from build123d import *

# Parameters (mm, degrees)
SKETCH1_R                    = 3.556
BOSS_EXTRUDE1_DEPTH          = 3.556
F_30_0_1285_DIAMETER_HOLE1_D = 3.2639
CHAMFER2_SIZE                = 0.381
F_65_0_035_DIAMETER_HOLE2_D  = 0.889
F_6_32_TAPPED_HOLE1_D        = 2.7051
F_6_32_TAPPED_HOLE1_DEPTH    = 5.7912
F_6_32_TAPPED_HOLE1_TIP      = 0.81269403


with BuildPart() as part:
    # Sketch1 → Boss-Extrude1 (new, symmetric)
    with BuildSketch(Plane(origin=(0, 0, 0), x_dir=(0, 0, -1), z_dir=(1, 0, 0))):
        Circle(SKETCH1_R)
    extrude(amount=BOSS_EXTRUDE1_DEPTH, both=True)

    # #30 (0.1285) Diameter Hole1 (through all)
    with Locations(Plane(origin=(3.556, 0, 0), x_dir=(0, 0, -1), z_dir=(1, 0, 0))):
        with Locations((0, 0)):
            Hole(F_30_0_1285_DIAMETER_HOLE1_D / 2)

    # Chamfer2
    chamfer2_edges = [part.edges().sort_by_distance(p)[0] for p in [
        (-3.556, 0, 3.556),
        (3.556, 0, 3.556),
    ]]
    chamfer(chamfer2_edges, length=CHAMFER2_SIZE)

    # #65 (0.035) Diameter Hole2 (through all)
    with Locations(Plane(origin=(0, 3.556, 0), x_dir=(1, 0, 0), z_dir=(0, 1, 0))):
        with Locations((0, 0)):
            Hole(F_65_0_035_DIAMETER_HOLE2_D / 2)

    # #6-32 Tapped Hole1
    with Locations(Plane(origin=(0, 3.556, 0), x_dir=(1, 0, 0), z_dir=(0, 1, 0))):
        with Locations((0, 0)):
            Hole(F_6_32_TAPPED_HOLE1_D / 2, depth=F_6_32_TAPPED_HOLE1_DEPTH)
            with Locations((0, 0, -(F_6_32_TAPPED_HOLE1_DEPTH + F_6_32_TAPPED_HOLE1_TIP / 2))):  # 118° drill point
                Cone(0, F_6_32_TAPPED_HOLE1_D / 2, F_6_32_TAPPED_HOLE1_TIP, mode=Mode.SUBTRACT)


solid = part.part
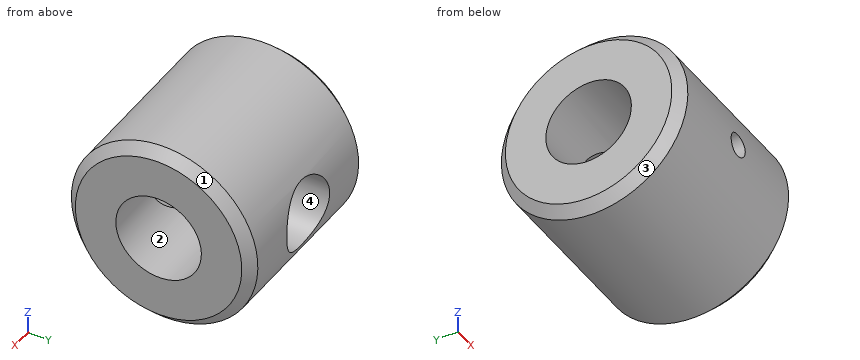
Here's how the part is built. I have some questions about the finished solid (model axes, mm). Face numbers are marked on the shaded views. Give positions to 0.01 mm unless a question says otherwise; leave off trailing zeros. Order: outer loops, then holes, each group sorted by start corner. A loop starts at its lowest first (then second) coordinate and runs counter-clockwise, first axis right, second up. Notation, with made-up numbers: M -21,19 L 19,19 A23 ccw 19,37 Z; hole C 49,77.25 d10. An arc over 180 degrees is marked long. Answer as a JSON object with one key per item and string values. Group by question number.
1) Please list where these lines run through material, in increasing order: L1, parallel to Z at x = 0, y = -1.6; L2, parallel to X at y = 2.75, z = -1; L3, parallel to Y at x = 1.75, z = 0. Write a range as [from, to].
2) Suppose I cut it at D-D, the plane x = 2.25. Write out the boundary of the cut face in (y, z).
3) I'm going to push flat-ended pins straight in: pin 1 Ø1 at (x, z) = (-0.5, 1) entering from +Y; pin 2 Ø4 at (y, z) = (0, 0) entering from -X; pin 3 Ø1.5 at (x, y) = (1, -1) entering from -Z; pin 4 Ø2 at (x, y) = (0.5, 2) entering from +Z. Where does each tip first touch, or does it pass through?
4) Suppose I cut it at A-A, the plane y = 0. Write out the boundary of the cut face in (x, z) (3 decimals).
5) Suppose I cut it at B-B, the plane z = 0. Write out the boundary of the cut face in (x, y) (1 decimal).
6) Suppose I cut it at C-C, the plane x = 0. Write out the boundary of the cut face in (y, z), plus the area to 3 significant figures.
7) We'd pull the mould along X, two halves only. Please class the marked faces 1, 2, 3 and 4: pulls with the +X half, pulls with the -X half, needs draft (parallel to the pull), parting line crosses it, or undercut.
Results found:
{
 "1": {"L1": "[-3.18, -1.35], [1.35, 3.18]", "L2": "[-3.56, -0.91], [0.91, 3.56]", "L3": "[-3.56, -1.63], [1.63, 3.56]"},
 "2": {"outline": "C 0,0 d7.11; hole C 0,0 d3.26"},
 "3": {"pin 1": "y = 3.44", "pin 2": "x = -3.56", "pin 3": "z = -3.55", "pin 4": "z = 3.41"},
 "4": {"outline": "M -3.556,-3.175 L -3.175,-3.556 L 3.175,-3.556 L 3.556,-3.175 L 3.556,-1.632 L -3.556,-1.632 Z; M -3.556,1.632 L 3.556,1.632 L 3.556,3.175 L 3.175,3.556 L -3.175,3.556 L -3.556,3.175 Z"},
 "5": {"outline": "M -3.6,-3.2 L -3.2,-3.6 L -0.4,-3.6 L -0.4,-2.8 L -1.4,-2.2 L -1.4,-1.6 L -3.6,-1.6 Z; M -3.6,1.6 L -1.4,1.6 L -1.4,3.6 L -3.2,3.6 L -3.6,3.2 Z; M 0.4,-3.6 L 3.2,-3.6 L 3.6,-3.2 L 3.6,-1.6 L 1.4,-1.6 L 1.4,-2.2 L 0.4,-2.8 Z; M 1.4,1.6 L 3.6,1.6 L 3.6,3.2 L 3.2,3.6 L 1.4,3.6 Z"},
 "6": {"outline": "M -3.53,-0.44 A3.56 ccw 3.29,-1.35 L 0.91,-1.35 A1.63 cw -0.91,-1.35 L -2.24,-1.35 L -2.78,-0.44 Z; M -3.53,0.44 L -2.78,0.44 L -2.24,1.35 L -0.91,1.35 A1.63 cw 0.91,1.35 L 3.29,1.35 A3.56 ccw Z", "area": "21.9 mm²"},
 "7": {"face 1": "pulls with the +X half", "face 2": "needs draft", "face 3": "pulls with the -X half", "face 4": "undercut"}
}
